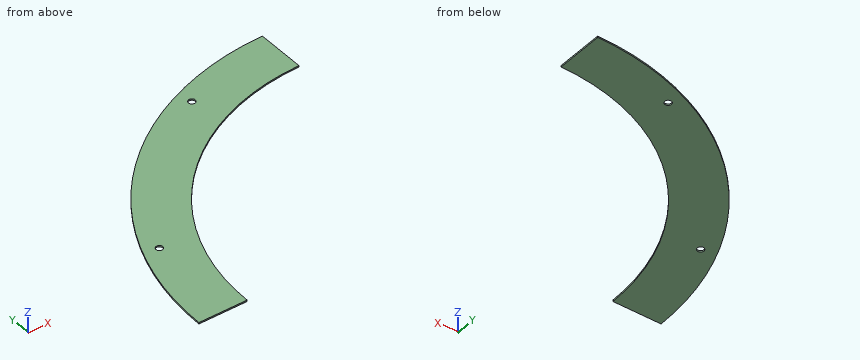
Autodesk Inventor part; units mm, degrees
ref_plane "YZ Plane" through (0, 0, 0) normal (1, 0, 0) x (0, 1, 0)
ref_plane "XZ Plane" through (0, 0, 0) normal (0, 1, 0) x (-1, 0, 0)
ref_plane "XY Plane" through (0, 0, 0) normal (0, 0, 1) x (1, 0, 0)
sketch "Sketch1" plane through (0, 0, 0) normal (0, 0, 1) x (1, 0, 0)
  arc A0 (0, 550) -> (-550, 0) centre (0, 0) ccw
  arc A1 (0, 450) -> (-450, 0) centre (0, 0) ccw
  line L0 (0, 550) -> (0, 450)
  line L1 (-450, 0) -> (-550, 0)
  point P0 (-500, 0)
  point P1 (0, 500)
  dimension "d0" = 1100
  dimension "d1" = 900
extrude "Plate1" add sketch "Sketch1" against normal blind 3
sketch "Sketch2" plane through (0, 0, 0) normal (0, 0, 1) x (1, 0, 0)
  line L0 (-550, 0) -> (-450, 0)
  arc A0 (0, 550) -> (-550, 0) centre (0, 0) ccw construction
  circle A1 centre (-480.4174, 198.9954) radius 7
  arc A2 (0, 450) -> (-450, 0) centre (0, 0) ccw construction
  circle A3 centre (0, 0) radius 520 construction
  line L1 (-480.4174, 198.9954) -> (0, 0) construction
  dimension "d11" = 1040
  dimension "d4" = 14
  dimension "d12" = 22.5
extrude "Cut1" cut sketch "Sketch2" against normal through all
pattern_circular "Circular Pattern1" count 2 over 45 about axis through (0, 0, 0) along (0, 0, -1) of "Cut1"
equation "\"d0\" = Диаметр_вн"
equation "\"d1\" = d0 - 2 * Ширина_кольца"
equation "\"d4\" = Диаметр_отв"
equation "\"d6\" = Thickness"
equation "\"d2\" = Thickness"
equation "\"BendReliefWidth\" = Thickness"
equation "\"BendReliefDepth\" = 0.5 * Thickness"
equation "\"CornerReliefSize\" = 4 * Thickness"
equation "\"MinimumRemnant\" = 2 * Thickness"
equation "\"TransitionRadius\" = BendRadius"
equation "\"JacobiRadiusSize\" = BendRadius"
equation "\"GapSize\" = Thickness"
properties part number "BSH 501 segment" material "Stainless Steel"
Model file for the job. Use its own axes, mm. Give positions to 0.01 mm unless a question says otherwise; leave off trailing zeros. Order: outer loops, then holes, each group sorted by start corner. A loop starts at its lowest first (then second) coordinate and runs counter-clockwise, first axis right, second up. Notation, with made-up numbers: M 20.5,49.5 L 75.5,49.5 A29 cw 75.5,87.5 Z; hole C 77.5,-20 d6. An arc over 180 degrees is marked long. Write item = value, one per line.
Q1. Cut at B-B, the plane y = 399. List the corners of the cut face in (x, z), then the cut area to 3 significant figures.
Derived:
outline = M -378.55,-3 L -208.08,-3 L -208.08,0 L -378.55,0 Z
area = 511 mm2
Q2. Flat gauge pin, fed straight in: pin 1 (4 mm diameter, centred on x = -489.5, y = 215.5, fed in from +Z). Where does the tip first touch, or does it go through?
Derived:
pin_1 = 0
Q3. Drill centre lines: line 1 (Y direction, x = -479.5, z = -2.8); line 2 (Y direction, x = -93, z = -2.25); line 3 (X direction, y = 242, z = -2.8). Where is each one in solid material? Low to high. Write a range as [from, to].
Derived:
line_1 = [0, 192.06], [205.94, 269.41]
line_2 = [440.29, 542.08]
line_3 = [-493.9, -379.39]
Q4. Cut at A-A, the plane z = -2.35. List the corners of the cut face in (x, y).
Derived:
outline = M -550,0 L -450,0 A450 cw 0,450 L 0,550 A550 ccw Z; hole C -480.42,199 d14; hole C -199,480.42 d14
Q5. Cut at C-C, the plane x = -263. List the corners of the cut face in (y, z).
Derived:
outline = M 365.15,-3 L 483.04,-3 L 483.04,0 L 365.15,0 Z
